The model under review builds one solid part; all positions refer to its coordinate system, in mm. A direction names the side the tool comes from. Give positions to 0.01 mm unless a question says otherwise; leave off trailing zeros. Loops run counter-clockwise (first coordinate to the right, second up) from the corner with the lowest first, then second, coordinate; pieces in that order, holes last. Notation, with made-up numbers: M 41,66 L 95,66 A30 cw 95,88 Z; hole C 75,71 d9. An arc over 180 degrees is marked long. Put each result on its own line as item: value. Start each with the question number.
Autodesk Inventor part; units mm, degrees
ref_plane "YZ Plane" through (0, 0, 0) normal (1, 0, 0) x (0, 1, 0)
ref_plane "XZ Plane" through (0, 0, 0) normal (0, 1, 0) x (-1, 0, 0)
ref_plane "XY Plane" through (0, 0, 0) normal (0, 0, 1) x (1, 0, 0)
sketch "Sketch1" plane through (0, 0, 0) normal (0, 0, 1) x (1, 0, 0)
  line L0 (0, 0) -> (90, 0)
  line L1 (90, 0) -> (90, 25)
  line L2 (90, 25) -> (60, 25)
  line L3 (60, 25) -> (60, 12)
  line L4 (60, 12) -> (35, 12)
  line L5 (35, 12) -> (35, 35)
  line L6 (0, 0) -> (0, 35)
  line L7 (17.5, 60) -> (0, 35)
  line L8 (17.5, 60) -> (35, 35)
  circle A0 centre (20, 20) radius 7
  dimension "d0" = 90
  dimension "d1" = 25
extrude "Extrusion1" add sketch "Sketch1" along normal blind 55
sketch "Sketch2" plane through (90, 0, 0) normal (1, 0, 0) x (0, 0, -1)
  line L0 (0, 25) -> (-55, 25)
  line L1 (-15, 25) -> (-55, 25)
  line L2 (-55, 35) -> (-55, 0)
  line L3 (-55, 5) -> (-15, 25)
  line L4 (-55, 25) -> (-55, 5)
  line L5 (-55, 12) -> (-55, 35)
  point P0 (0, 0)
extrude "Extrusion2" cut sketch "Sketch2" against normal blind 20
sketch "Sketch3" plane through (35, 12, 0) normal (1, 0, 0) x (0, 0, -1)
  line L0 (0, 48) -> (-55, 48)
  line L1 (-15, 48) -> (-15, 30)
  line L2 (0, 23) -> (-55, 23)
  line L3 (-15, 30) -> (-40, 30)
  line L4 (-40, 30) -> (-40, 48)
  line L5 (-15, 48) -> (-40, 48)
  point P0 (0, -12)
  dimension "d6" = 18
extrude "Extrusion3" cut sketch "Sketch3" against normal blind 35
properties part number "P4-10"
(1) We need section C-C, the plane y = 20. Write out the cut boundary in (x, z), plus the area to 4 significant figures.
(2) To check wall thickness, follow L1, parallel to Y at x = 20, z = 26; L2, parallel to Y at x = 51, z = 9.5; L3, parallel to X at y = 17.5, z = 23.5. State the ranges of each line that lie inside material, in increasing order. Write a range as [from, to].
(3) Insertion check: pin 1 (10 mm diameter, centred on x = 60.5, z = 39.5, fed in from -Y); pin 2 (11 mm diameter, centred on x = 20, y = 20, fed in from -Z); pin 3 (1 mm diameter, centred on x = 65, z = 33, fed in from +Y); pin 4 (11.5 mm diameter, centred on y = 27.5, z = 39.5, fed in from +X). Each pin has a flat end and moves straight along its axis. Give the tip position at first contact, or say it passes through.
(4) We need section B-B, the plane z = 23.5. Write out the cut boundary in (x, y), plus the area to 3 significant figures.
(5) We need section D-D, the plane x = 20. Write out the cut boundary in (y, z).
(6) We need section A-A, the plane y = 47. Write out the cut boundary in (x, z), plus the area to 3 significant figures.
(7) For faces 5 (the flat face through (18, 42, 27)), 6 (the flat face through (80, 15, 35)), 7 (the flat face through (60, 19, 27)), 8 (the flat face through (69, 25, 21)), list the 3-axis set-ups (+Z, -Z, +X, -X, +Y, -Y) from which the entire face can be reached by the end or side of a thin tool; tool diameter is ignored.
(8) Draft analysis for pull direction Z (two halves, no side actions). For faces 1 (the flat face through (34, 17, 55)), 2 (the flat face through (18, 49, 40)), 3 (the flat face through (18, 49, 15)), 4 (the flat face through (44, 0, 27)), state which applies: +Z half, -Z half, draft (parallel to the pull), parting line (faces both ways), or undercut.
Check sheet entries:
1. outline: M 0,0 L 13,0 L 13,55 L 0,55 Z; M 27,0 L 35,0 L 35,55 L 27,55 Z; M 60,0 L 90,0 L 90,25 L 70,25 L 70,55 L 60,55 Z
1. area: 2,205 mm²
2. L1: y = [0, 13], [27, 42]
2. L2: y = [0, 12]
2. L3: x = [0, 13.46], [26.54, 35], [60, 90]
3. pin 1: stops at y = 0
3. pin 2: passes through
3. pin 3: stops at y = 25
3. pin 4: stops at x = 70
4. outline: M 0,0 L 90,0 L 90,20.75 L 70,20.75 L 70,25 L 60,25 L 60,12 L 35,12 L 35,35 L 30.1,42 L 4.9,42 L 0,35 Z; hole C 20,20 d14
4. area: 2,250 mm²
5. outline: M 0,0 L 13,0 L 13,55 L 0,55 Z; M 27,0 L 56.43,0 L 56.43,15 L 42,15 L 42,40 L 56.43,40 L 56.43,55 L 27,55 Z
6. outline: M 8.4,0 L 26.6,0 L 26.6,15 L 8.4,15 Z; M 8.4,40 L 26.6,40 L 26.6,55 L 8.4,55 Z
6. area: 546 mm²
7. face 5: +X, -X, +Y
7. face 6: +Z, +X, +Y
7. face 7: +Z, -Z, +Y
7. face 8: +Z, -Z, +X, +Y
8. face 1: +Z half
8. face 2: undercut
8. face 3: undercut
8. face 4: draft
